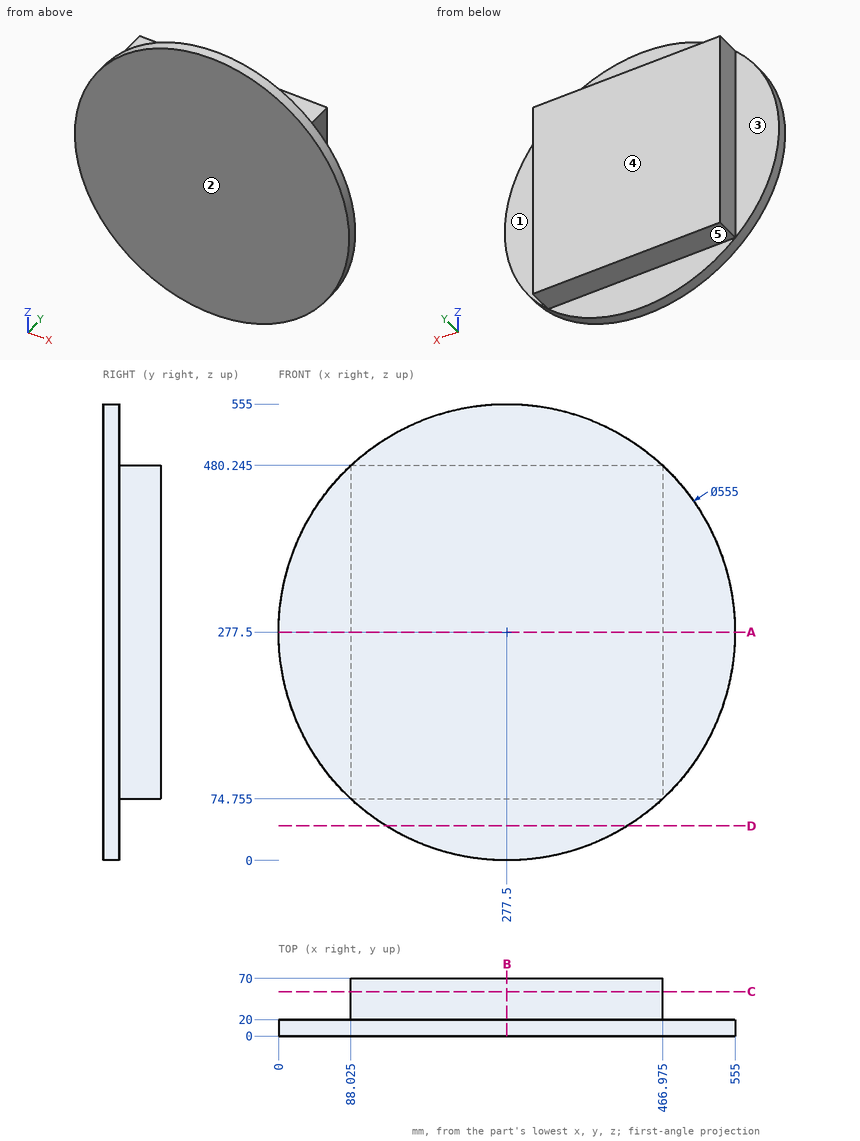
Could you check a few things on this drawing? It's one solid part, dimensions in mm from its lowest x, y, z. A direction names the side the tool comes from. Give positions to 0.01 mm unless a question says otherwise; leave off trailing zeros. Loops run counter-clockwise (first coordinate to the right, second up) from the corner with the lowest first, then second, coordinate; pieces in that order, holes last. Notation, with made-up numbers: M 35.25,81 L 82.25,81 A19 cw 82.25,114 Z; hole C -30,-32.5 d5. An arc over 180 degrees is marked long. Return JSON: item names as keys, results as strings.
Item 1: On a 3-axis mill with a long thin cutter (end or side, diameter ignored), from which of +Z, -Z, +X, -X, +Y, -Y can I reach the whole of each face in a straight line? I mean the marked faces 1, 2, 3, 4 and 5. Say none if no direction works.
A:
{"face 1": "+Z, -Z, +X, +Y", "face 2": "+Z, -Z, +X, -X, -Y", "face 3": "+Z, -Z, -X, +Y", "face 4": "+Z, -Z, +X, -X, +Y", "face 5": "-Z, +X, -X, +Y"}
Item 2: Imagine slicing it at C-C on y = 54. List the corners of the cut face in (x, z) for me (1 decimal), then the cut area to 3 significant figures.
A:
{"outline": "M 88,74.8 L 467,74.8 L 467,480.2 L 88,480.2 Z", "area": "154,000 mm^2"}
Item 3: Please list where these lines run through material, in increasing order: line 1 (Z direction, x = 213, y = 53) (1 decimal); line 2 (Y direction, x = 520, z = 375); line 3 (X direction, y = 51, z = 89) (1 decimal).
A:
{"line 1": "z = 74.8 to 480.2", "line 2": "y = 0 to 20", "line 3": "x = 88 to 467"}
Item 4: Imagine slicing it at A-A on z = 277.5. List the corners of the cut face in (x, y) for me (1 decimal), then the cut area to 3 significant figures.
A:
{"outline": "M 0,0 L 555,0 L 555,20 L 467,20 L 467,70 L 88,70 L 88,20 L 0,20 Z", "area": "30,000 mm^2"}
Item 5: I'm going to push flat-ended pins straight in: pin 1 Ø6 at (x, y) = (261, 36.5) entering from +Z (1 decimal); pin 2 Ø3 at (y, z) = (28, 455) entering from +X (1 decimal); pin 3 Ø5 at (x, y) = (232.5, 60) entering from -Z (1 decimal); pin 4 Ø3 at (x, z) = (291.5, 323) entering from -Y. Where does each tip first touch, or does it pass through?
A:
{"pin 1": "stops at z = 480.2", "pin 2": "stops at x = 467", "pin 3": "stops at z = 74.8", "pin 4": "stops at y = 0"}
Item 6: Imagine slicing it at D-D on z = 42. List the corners of the cut face in (x, y) for me (1 decimal), then the cut area to 3 significant figures.
A:
{"outline": "M 130.7,0 L 424.3,0 L 424.3,20 L 130.7,20 Z", "area": "5,870 mm^2"}
Item 7: Imagine slicing it at B-B on x = 277.5. List the corners of the cut face in (y, z) for me (1 decimal), then the cut area to 3 significant figures.
A:
{"outline": "M 0,0 L 20,0 L 20,74.8 L 70,74.8 L 70,480.2 L 20,480.2 L 20,555 L 0,555 Z", "area": "31,400 mm^2"}
